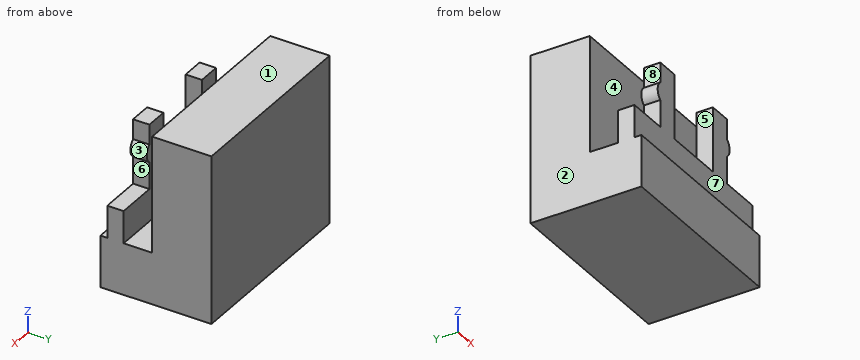
Autodesk Inventor part; units mm, degrees
ref_plane "YZ Plane" through (0, 0, 0) normal (1, 0, 0) x (0, 1, 0)
ref_plane "XZ Plane" through (0, 0, 0) normal (0, 1, 0) x (-1, 0, 0)
ref_plane "XY Plane" through (0, 0, 0) normal (0, 0, 1) x (1, 0, 0)
sketch "Sketch1" plane through (0, 0, 0) normal (0, 0, 1) x (1, 0, 0)
  line L0 (-6.3366, 6.9163) -> (21.6034, 6.9163)
  line L1 (21.6034, 6.9163) -> (21.6034, -8.3237)
  line L2 (21.6034, -8.3237) -> (-6.3366, -8.3237)
  line L3 (-6.3366, -8.3237) -> (-6.3366, 6.9163)
  point P0 (0, 0)
  dimension "d0" = 27.94
  dimension "d1" = 15.24
extrude "Extrusion1" add sketch "Sketch1" along normal blind 7.62
sketch "Sketch2" plane through (0, 0, 7.62) normal (0, 0, 1) x (1, 0, 0)
  line L0 (-6.3366, 6.9163) -> (-6.3366, -8.3237)
  line L1 (21.6034, -8.3237) -> (21.6034, 6.9163)
  line L2 (21.6034, 0.3123) -> (21.6034, 2.7253)
  line L3 (-6.3366, 2.7253) -> (-6.3366, 0.3123)
  line L4 (21.6034, 6.9163) -> (-6.3366, 6.9163)
  line L5 (-6.3366, -8.3237) -> (21.6034, -8.3237)
  line L6 (0.9631, 2.7253) -> (-0.2406, 2.7253)
  line L7 (-0.2406, 0.3123) -> (0.9631, 0.3123)
  line L8 (-0.2406, 0.3123) -> (-0.2406, 2.7253)
  line L9 (-0.2406, 0.3123) -> (3.0821, 0.3123)
  line L10 (3.0821, 0.3123) -> (3.0821, 2.7253)
  line L11 (3.0821, 2.7253) -> (-0.2406, 2.7253)
  line L12 (-0.2406, 2.7253) -> (-0.2406, 0.3123)
  line L13 (14.3038, 2.7253) -> (15.5074, 2.7253)
  line L14 (15.5074, 0.3123) -> (14.3038, 0.3123)
  line L15 (15.5074, 0.3123) -> (15.5074, 2.7253)
  line L16 (15.5074, 0.3123) -> (12.1847, 0.3123)
  line L17 (12.1847, 0.3123) -> (12.1847, 2.7253)
  line L18 (12.1847, 2.7253) -> (15.5074, 2.7253)
  line L19 (15.5074, 2.7253) -> (15.5074, 0.3123)
  line L20 (-6.3366, -0.7037) -> (21.6034, -0.7037)
  line L21 (-6.3366, 2.7253) -> (21.6034, 2.7253)
  line L22 (21.6034, 2.7253) -> (21.6034, 0.3123)
  line L23 (21.6034, 0.3123) -> (-6.3366, 0.3123)
  line L24 (-6.3366, 0.3123) -> (-6.3366, 2.7253)
  point P0 (0, 0)
  point P1 (-0.2406, 1.5188)
  point P2 (15.2669, 0)
  point P3 (15.5074, 1.5188)
  dimension "d6" = 6.096
extrude "Extrusion2" add sketch "Sketch2" along normal blind 8.7376 contours L6 L11 L10 L9 L7 L8 | L15 L14 L16 L17 L18 L13
sketch "Sketch3" plane through (-0.2406, 2.7253, 7.62) normal (0, 1, 0) x (1, 0, 0)
  line L0 (3.3227, -8.7376) -> (0, -8.7376)
  line L1 (3.3227, -11.3552) -> (0, -11.3552)
  line L2 (0, -11.3552) -> (0, -8.7376)
  line L3 (3.3227, -8.7376) -> (0, -8.7376)
  line L4 (-6.096, 7.62) -> (21.844, 7.62)
  line L5 (3.3227, -11.3552) -> (3.3227, -8.7376)
  arc A0 (0, -8.7376) -> (0, -11.3552) centre (1.0363, -10.0464) ccw
  line L6 (12.4253, -8.7376) -> (15.748, -8.7376)
  line L7 (12.4253, -11.3552) -> (15.748, -11.3552)
  line L8 (15.748, -11.3552) -> (15.748, -8.7376)
  line L9 (12.4253, -8.7376) -> (15.748, -8.7376)
  line L10 (12.4253, -11.3552) -> (12.4253, -8.7376)
  arc A1 (15.748, -11.3552) -> (15.748, -8.7376) centre (14.7117, -10.0464) ccw
  point P0 (0.2406, 7.62)
extrude "Extrusion3" add sketch "Sketch3" against normal up to surface (2.413 mm away)
extrude "Extrusion4" add sketch "Sketch2" along normal blind 14.2875 contours L6 L11 L10 L9 L7 L8 | L15 L14 L16 L17 L18 L13
sketch "Sketch4" plane through (-6.3366, 6.9163, 0) normal (0, 1, 0) x (1, 0, 0)
  point P0 (6.3366, 0)
sketch "Sketch5" plane through (0, 0, 7.62) normal (0, 0, 1) x (1, 0, 0)
  line L0 (21.6034, 6.9163) -> (-6.3366, 6.9163)
  line L1 (-6.3366, 15.6735) -> (21.6034, 15.6735)
  line L2 (21.6034, 15.6735) -> (21.6034, 6.9163)
  line L3 (21.6034, 6.9163) -> (-6.3366, 6.9163)
  line L4 (-6.3366, 6.9163) -> (-6.3366, 15.6735)
  point P0 (0, 0)
extrude "Extrusion5" add sketch "Sketch5" along normal blind 17.145 and the other way blind 7.62
extrude "Extrusion6" cut sketch "Sketch2" against normal blind 25.4 contours L20 L1 L5 L0
extrude "Extrusion7" add sketch "Sketch2" along normal blind 4.7625 contours L21 L8 L23 L0 | L1 L23 L15 L21 | L21 L17 L23 L10
properties part number "Attachment2"
Verification items for the finished model (mm, model axes). Face numbers are marked on the shaded views. A direction names the side the tool comes from. Round coordinates to 2 decimals unless told otherwise and drop trailing zeros. Write each loop counter-clockwise with the first axis right and the second up, starting at its lowest first coordinate (ties: lowest second). Pieces come first, ordered by that corner, then holes. Notation, with made-up numbers: (77, 80.25) -> (113, 80.25) arc R32 cw to (113, 110.25) -> close; hole circle Ø6 at (30, 79.25). An arc over 180 degrees is marked (long way). Write each question's results on one line, items separated by ' | '.
Q1. Draft check along Z on the marked faces 1, 2 and 3. Enter one of: released by +Z, released by -Z, zero draft, split by the parting line, or undercut.
Derived:
face 1: released by +Z | face 2: zero draft | face 3: undercut
Q2. Access from +Z, -Z, +X, -X, +Y, -Y to the whole of each face (thin tool, end or side, straight path). Record for the marked faces 4, 5, 6, 7 and 8.
Derived:
face 4: +Z, +X, -X | face 5: +Z, -Y | face 6: +X, -Y | face 7: +Z, +X, -X, -Y | face 8: +Z, -X, -Y
Q3. Sectioned sample at C-C, the plane x = 4.5. Record the boundary of the cut face in (y, z) (1 decimal), and give its area (3 significant figures).
Derived:
outline: (-0.7, 0) -> (15.7, 0) -> (15.7, 24.8) -> (6.9, 24.8) -> (6.9, 7.6) -> (2.7, 7.6) -> (2.7, 12.4) -> (0.3, 12.4) -> (0.3, 7.6) -> (-0.7, 7.6) -> close | area: 286 mm²
Q4. Sectioned sample at B-B, the plane z = 20. Record the boundary of the cut face in (x, y).
Derived:
outline: (-6.34, 6.92) -> (21.6, 6.92) -> (21.6, 15.67) -> (-6.34, 15.67) -> close; (-0.24, 0.31) -> (3.08, 0.31) -> (3.08, 2.73) -> (-0.24, 2.73) -> close; (12.18, 0.31) -> (15.51, 0.31) -> (15.51, 2.73) -> (12.18, 2.73) -> close
Q5. Sectioned sample at A-A, the plane z = 8. Record the boundary of the cut face in (x, y), and give its area (3 significant figures).
Derived:
outline: (-6.34, 0.31) -> (21.6, 0.31) -> (21.6, 2.73) -> (-6.34, 2.73) -> close; (-6.34, 6.92) -> (21.6, 6.92) -> (21.6, 15.67) -> (-6.34, 15.67) -> close | area: 312 mm²
Q6. Thickness scan on probe 1 along Y at (x, z) = (19.5, 9.75); probe 2 along Z at (x, y) = (17.75, 4.75); probe 3 along Y at (x, z) = (12, 15.5). Record the ranges inside material, lowest first.
Derived:
probe 1: y = 0.31 to 2.73, 6.92 to 15.67 | probe 2: z = 0 to 7.62 | probe 3: y = 6.92 to 15.67
Q7. Sectioned sample at D-D, the plane y = 2. Record the boundary of the cut face in (x, z), and give its area (3 significant figures).
Derived:
outline: (-6.34, 0) -> (21.6, 0) -> (21.6, 12.38) -> (15.51, 12.38) -> (15.51, 16.36) arc R1.67 ccw to (15.51, 18.98) -> (15.51, 21.91) -> (12.18, 21.91) -> (12.18, 12.38) -> (3.08, 12.38) -> (3.08, 21.91) -> (-0.24, 21.91) -> (-0.24, 18.98) arc R1.67 ccw to (-0.24, 16.36) -> (-0.24, 12.38) -> (-6.34, 12.38) -> close | area: 412 mm²
Q8. Go/stop test with flat-tipped pins: pin 1 Ø2 at (y, z) = (1.5, 19) entering from -X; pin 2 Ø1.2 at (y, z) = (2, 15) entering from +X; pin 3 Ø1.5 at (x, y) = (2, 11) entering from -Z; pin 4 Ø1.9 at (y, z) = (1.5, 21) entering from -X. Record where each tip stops, or that it passes through.
Derived:
pin 1: stops at x = -0.84 | pin 2: stops at x = 15.51 | pin 3: stops at z = 0 | pin 4: stops at x = -0.24
